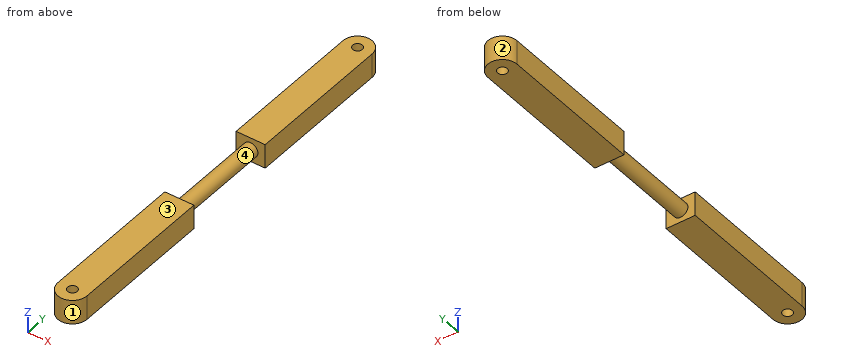
from build123d import *

# Parameters (mm, degrees)
SKETCH_1_R          = 1
EXTRUDE_1_DEPTH     = 2.5
SKETCH_4_R          = 5.341815289
SKETCH_4_R_2        = 1.5
CUT_EXTRUDE_2_DEPTH = 10


with BuildPart() as part:
    # 草图1 → 凸台-拉伸1 (new, symmetric)
    with BuildSketch(Plane.XY):
        with BuildLine():
            Line((3, 0), (3, -80))
            ThreePointArc((3, -80), (0, -83), (-3, -80))
            Line((-3, -80), (-3, 0))
            ThreePointArc((-3, 0), (0, 3), (3, 0))
        make_face()
        Circle(SKETCH_1_R, mode=Mode.SUBTRACT)
        with Locations((0, -80)):
            Circle(SKETCH_1_R, mode=Mode.SUBTRACT)
    extrude(amount=EXTRUDE_1_DEPTH, both=True)


with BuildPart() as part_1:
    # Move Body 1: moved
    add(part.part.moved(Location((0, 40, 0))))

    # 草图4 → 切除-拉伸2 (cut, symmetric)
    with BuildSketch(Plane(origin=(0, 0, 0), x_dir=(1, 0, 0), z_dir=(0, 1, 0))):
        Circle(SKETCH_4_R)
        with Locations(Location((0, 0, 0), (0, 0, 270))):
            Circle(SKETCH_4_R_2, mode=Mode.SUBTRACT)
    extrude(amount=CUT_EXTRUDE_2_DEPTH, both=True, mode=Mode.SUBTRACT)


solid = part_1.part
Verification items for the finished model (mm, model axes). Face numbers are marked on the shaded views. Give positions to 0.01 mm unless a question says otherwise; leave off trailing zeros. Order: outer loops, then holes, each group sorted by start corner. A loop starts at its lowest first (then second) coordinate and runs counter-clockwise, first axis right, second up. Notation, with made-up numbers: M -11.75,-25.75 L 0.25,-25.75 A7 cw 0.25,-16.75 Z; hole C 53,46.25 d5. An arc over 180 degrees is marked long. Answer as a JSON object with one key per item and string values. Group by question number.
1) Cross-section at A-A (x = 0). Enter the section's corners in (y, z).
2) Mould release check, pull along Y, two halves, no side actions. Record for the marked faces 1, 2, 3 and 4: released by +Y, released by -Y, zero draft, split by the parting line, or undercut.
3) Depth check by flat-ended pin: pin 1 Ø1.5 at (x, z) = (-1, -0.5) entering from -Y. Enter the tip coordinate at first touch or a pass-through.
4) Scan lines: line 1 along Y through (x, z) = (0, -1.4); line 2 along X through (y, z) = (-40, -1.35); line 3 along Y through (x, z) = (-0.8, 2.2). Record each from-to range of solid material in increasing order. Write a range as [from, to].
5) Cross-section at B-B (z = 0). Enter the section's corners in (x, y), then the cut area to 3 significant figures.
Result sheet:
{
 "1": {"outline": "M -43,-2.5 L -41,-2.5 L -41,2.5 L -43,2.5 Z; M -39,-2.5 L -10,-2.5 L -10,-1.5 L 10,-1.5 L 10,-2.5 L 39,-2.5 L 39,2.5 L 10,2.5 L 10,1.5 L -10,1.5 L -10,2.5 L -39,2.5 Z; M 41,-2.5 L 43,-2.5 L 43,2.5 L 41,2.5 Z"},
 "2": {"face 1": "released by -Y", "face 2": "released by +Y", "face 3": "zero draft", "face 4": "undercut"},
 "3": {"pin 1": "stops at y = -42.99"},
 "4": {"line 1": "y = [-43, -41], [-39, 39], [41, 43]", "line 2": "x = [-3, -1], [1, 3]", "line 3": "y = [-42.89, -40.6], [-39.4, -10], [10, 39.4], [40.6, 42.89]"},
 "5": {"outline": "M -3,-40 A3 ccw 3,-40 L 3,-10 L 1.5,-10 L 1.5,10 L 3,10 L 3,40 A3 ccw -3,40 L -3,10 L -1.5,10 L -1.5,-10 L -3,-10 Z; hole C 0,-40 d2; hole C 0,40 d2", "area": "442 mm2"}
}
